Source: CAD feature listing. Evaluate the final solid. Frame: model axes, mm. A direction names the side the tool comes from. Give positions to 0.01 mm unless a question says otherwise; leave off trailing zeros. Order: outer loops, then holes, each group sorted by start corner. A loop starts at its lowest first (then second) coordinate and runs counter-clockwise, first axis right, second up.
```python
from build123d import *

# Parameters (mm, degrees)
F0_W     = 420
F0_H     = 100
F1_DEPTH = 15
F2_R     = 20
F3_DEPTH = 15.001
F4_R     = 20.670136
F5_DEPTH = 25


with BuildPart() as f1:
    # F0 (on Front) → F1 (new body)
    with BuildSketch(Plane.XZ):
        Rectangle(F0_W, F0_H)
    extrude(amount=F1_DEPTH)

    # F2 (on face) → F3 (cut, through all)
    with BuildSketch(Plane.XZ.offset(15)):
        with Locations((-165, 15)):
            Circle(F2_R)
    extrude(amount=-F3_DEPTH, mode=Mode.SUBTRACT)

    # F4 (on face) → F5 (join)
    with BuildSketch(Plane.XZ.offset(15)):
        with Locations((62.055632, 0)):
            Circle(F4_R)
    extrude(amount=F5_DEPTH)


solid = f1.part
```
1) Pin query (flat end, axial travel): pin 1 (1 mm diameter, centred on x = 149.5, z = -29, fed in from -Y); pin 2 (2 mm diameter, centred on x = 135.5, z = 2, fed in from +Y). Return the tip coordinate at first contact, or that it passes through.
Report:
pin 1: stops at y = -15
pin 2: stops at y = 0
2) Material intervals for L1, parallel to Z at x = -165, y = -3.5; L2, parallel to Y at x = -107, z = 18; L3, parallel to Z at x = -169.5, y = -5.5, sorted ascending.
Report:
L1: z = -50 to -5, 35 to 50
L2: y = -15 to 0
L3: z = -50 to -4.49, 34.49 to 50
3) Section query A-A, the plane y = -11.5. Return the cut outline in (x, z), and give its area (3 significant figures).
Report:
outline: (-210, -50) - (210, -50) - (210, 50) - (-210, 50) - close; hole circle Ø40 at (-165, 15)
area: 40,700 mm2
4) Section query C-C, the plane z = 0. Return the cut outline in (x, y).
Report:
outline: (-210, -15) - (-178.23, -15) - (-178.23, 0) - (-210, 0) - close; (-151.77, -15) - (41.39, -15) - (41.39, -40) - (82.73, -40) - (82.73, -15) - (210, -15) - (210, 0) - (-151.77, 0) - close
5) Section query B-B, the plane x = -165. Return the cut outline in (y, z).
Report:
outline: (-15, -50) - (0, -50) - (0, -5) - (-15, -5) - close; (-15, 35) - (0, 35) - (0, 50) - (-15, 50) - close
6) Draft query along Z for faces 1 (the flat face through (-3, -7, -50)), 2 (the flat face through (62, -40, 0)), 3 (the cylindrical face through (-184.98, -7.6, 15.88)). Return one class per face: +Z half, -Z half, draft (parallel to the pull), parting line (faces both ways), or undercut.
Report:
face 1: -Z half
face 2: draft
face 3: undercut
7) Section query D-D, the plane x = -95. Return the cut outline in (y, z), and give its area (3 significant figures).
Report:
outline: (-15, -50) - (0, -50) - (0, 50) - (-15, 50) - close
area: 1,500 mm2
8) Reachability of faces 4 (the cylindrical face through (41.405, -27.325, 0.909)), 5 (the flat face through (-3, 0, 1)) from +Z, -Z, +X, -X, +Y, -Y: full face, straight path, thin tool, end or side. Return the list, or none.
Report:
face 4: -Y
face 5: +Z, -Z, +X, -X, +Y
